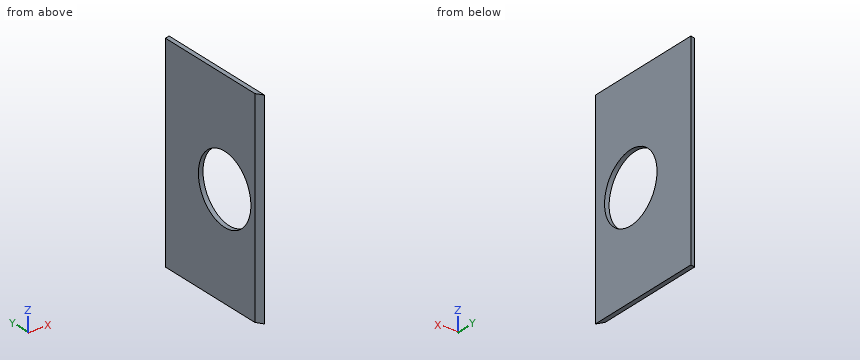
from build123d import *

# Parameters (mm, degrees)
AUFSATZ_LINEAR_AUSTRAGEN1_DEPTH  = 450
F_15_0_15_DURCHMESSER_BOHRUNG1_D = 150


with BuildPart() as part:
    # Skizze1 → Aufsatz-Linear austragen1 (new body)
    with BuildSketch(Plane.XY):
        Polygon((331.858259494, 76.52367356), (341.858259494, 78.794563683), (341.858259494, -194.367647059), (331.858259494, -179.367647059), align=None)
    extrude(amount=AUFSATZ_LINEAR_AUSTRAGEN1_DEPTH)

    # Ø15.0 (15) Durchmesser Bohrung1 (through all)
    with Locations(Plane(origin=(331.858259494, -93.067647059, 225), x_dir=(0, -1, 0), z_dir=(-1, 0, 0))):
        with Locations((0, 0)):
            Hole(F_15_0_15_DURCHMESSER_BOHRUNG1_D / 2)


solid = part.part
CAD build for the part. Positions are in the model's coordinates, mm. Give positions to 0.01 mm unless a question says otherwise; leave off trailing zeros. Order: outer loops, then holes, each group sorted by start corner. A loop starts at its lowest first (then second) coordinate and runs counter-clockwise, first axis right, second up. Notation, with made-up numbers: (-37.5, 42.5) - (-25.5, 42.5) arc R24 cw to (-25.5, 64.5) - close; hole circle Ø2 at (57, 43.25). An arc over 180 degrees is marked (long way). Answer in a Markdown table with one row per item.
1. Saw through at D-D, the plane z = 56. Give the cut face in (x, y), plus the area to 3 significant figures.
Data:
| item | result |
|---|---|
| outline | (331.86, -179.37) - (341.86, -194.37) - (341.86, 78.79) - (331.86, 76.52) - close |
| area | 2,650 mm² |
2. Saw through at A-A, the plane z = 225. Give the cut face in (x, y).
Data:
| item | result |
|---|---|
| outline | (331.86, -179.37) - (341.86, -194.37) - (341.86, -168.07) - (331.86, -168.07) - close; (331.86, -18.07) - (341.86, -18.07) - (341.86, 78.79) - (331.86, 76.52) - close |
3. Flat gauge pins, fed straight in: pin 1 (5 mm diameter, centred on x = 337.5, z = 179.5, fed in from -Y); pin 2 (4 mm diameter, centred on x = 338.5, z = 328, fed in from -Y); pin 3 (4 mm diameter, centred on x = 334.5, z = 374.5, fed in from -Y). Where does each tip first touch, or does it go through?
Data:
| item | result |
|---|---|
| pin 1 | stops at y = -191.58 |
| pin 2 | stops at y = -192.33 |
| pin 3 | stops at y = -186.33 |
4. Probe probe 1 along Z at (x, y) = (339.25, -94); probe 2 along Y at (x, z) = (334, 253.5); probe 3 along Z at (x, y) = (339, -57.5). List the from-to ranges inside material, lowest first. Write a range as [from, to].
Data:
| item | result |
|---|---|
| probe 1 | z = [0, 150.01], [299.99, 450] |
| probe 2 | y = [-182.58, -162.44], [-23.69, 77.01] |
| probe 3 | z = [0, 158.97], [291.03, 450] |
5. Saw through at B-B, the plane y = -47. Give the cut face in (x, z).
Data:
| item | result |
|---|---|
| outline | (331.86, 0) - (341.86, 0) - (341.86, 165.82) - (331.86, 165.82) - close; (331.86, 284.18) - (341.86, 284.18) - (341.86, 450) - (331.86, 450) - close |
6. Saw through at C-C, the plane x = 333.5. Give the cut face in (y, z), plus the area to 3 significant figures.
Data:
| item | result |
|---|---|
| outline | (-181.83, 0) - (76.9, 0) - (76.9, 450) - (-181.83, 450) - close; hole circle Ø150 at (-93.07, 225) |
| area | 98,800 mm² |
